Read the model definition and answer for the solid it produces. Units are mm, in the model's axes. A direction names the side the tool comes from. Give positions to 0.01 mm unless a question says otherwise; leave off trailing zeros. Write each loop counter-clockwise with the first axis right and the second up, starting at its lowest first coordinate (ties: lowest second). Pieces come first, ordered by that corner, then holes. Notation, with made-up numbers: M -5.5,-38 L 51.5,-38 A26 cw 51.5,-19 Z; hole C -25,10.25 d3. An arc over 180 degrees is marked long. Put each result on its own line as item: value.
from build123d import *

# Parameters (mm, degrees)
SKETCH2_W           = 38.1
SKETCH2_H           = 50.8
SKETCH2_R           = 13.335
BOSS_EXTRUDE2_DEPTH = 3.175
SKETCH4_W           = 38.1
SKETCH4_H           = 50.8
SKETCH4_R           = 13.335
BOSS_EXTRUDE3_DEPTH = 3.175
BOSS_EXTRUDE4_DEPTH = 127
CUT_EXTRUDE3_DEPTH  = 127
BOSS_EXTRUDE7_DEPTH = 127
SKETCH16_R          = 38.1
BOSS_EXTRUDE8_DEPTH = 25.4
CUT_EXTRUDE6_REACH  = 522.886
SKETCH19_W          = 33.866666667
SKETCH19_H          = 115.824
SKETCH19_W_2        = 33.866666666
CUT_EXTRUDE7_DEPTH  = 34.925


with BuildPart() as part:
    # Sketch2 → Boss-Extrude2 (new, symmetric)
    with BuildSketch(Plane(origin=(63.5, 0, 0), x_dir=(0, 0, -1), z_dir=(1, 0, 0))):
        Rectangle(SKETCH2_W, SKETCH2_H)
        Circle(SKETCH2_R, mode=Mode.SUBTRACT)
    extrude(amount=BOSS_EXTRUDE2_DEPTH, both=True)



with BuildPart() as body_2:
    # Sketch4 → Boss-Extrude3 (new, symmetric)
    with BuildSketch(Plane(origin=(292.1, 0, -263.652), x_dir=(0, 0, 1), z_dir=(-1, 0, 0))):
        with Locations((263.652, 0)):
            Rectangle(SKETCH4_W, SKETCH4_H)
        with Locations(Location((263.652, 0, 0), (0, 0, 180))):
            Circle(SKETCH4_R, mode=Mode.SUBTRACT)
    extrude(amount=BOSS_EXTRUDE3_DEPTH, both=True)


with BuildPart() as part_1:
    add(part.part)

    add(body_2.part)  # Boss-Extrude4 merges body 2
    # Sketch6 → Boss-Extrude4 (add, symmetric)
    with BuildSketch(Plane(origin=(177.8, 0, 0), x_dir=(0, 0, -1), z_dir=(1, 0, 0))):
        Polygon((-19.05, -25.4), (-61.976, -25.4), (-61.976, -255.524), (236.474, -255.524), (236.474, -217.424), (134.874, -25.4), (19.05, -25.4), align=None)
    extrude(amount=BOSS_EXTRUDE4_DEPTH, both=True)

    # Sketch13 → Cut-Extrude3 (cut, symmetric)
    with BuildSketch(Plane(origin=(177.8, 0, 0), x_dir=(0, 0, -1), z_dir=(1, 0, 0))):
        Polygon((-52.451, -34.925), (129.137596743, -34.925), (226.949, -219.788552156), (226.949, -255.524), (-61.976, -255.524), (-61.976, -219.788552156), (-52.451, -219.788552156), align=None)
    extrude(amount=CUT_EXTRUDE3_DEPTH, both=True, mode=Mode.SUBTRACT)

    # Sketch14 → Boss-Extrude7 (add, symmetric)
    with BuildSketch(Plane(origin=(177.8, 0, 0), x_dir=(0, 0, -1), z_dir=(1, 0, 0))):
        Polygon((226.949, -219.788552156), (-52.451, -219.788552156), (-52.451, -210.263552156), (221.90931746, -210.263552156), align=None)
        Polygon((-52.451, -146.763552156), (188.311433862, -146.763552156), (183.271751323, -137.238552156), (-52.451, -137.238552156), align=None)
    extrude(amount=BOSS_EXTRUDE7_DEPTH, both=True)

    # Sketch16 → Boss-Extrude8 (add)
    with BuildSketch(Plane(origin=(304.8, 0, 0), x_dir=(0, 0, -1), z_dir=(1, 0, 0))):
        with Locations(Location((-23.876, -232.488552156, 0), (0, 0, 160.528779366))):
            Circle(SKETCH16_R)
        with Locations(Location((160.274, -232.488552156, 0), (0, 0, 160.528779366))):
            Circle(SKETCH16_R)
    boss_extrude8 = extrude(amount=BOSS_EXTRUDE8_DEPTH)

    # Mirror1: Boss-Extrude8 across plane
    add(boss_extrude8.mirror(Plane(origin=(177.8, 0, 0), x_dir=(0, 0, 1), z_dir=(1, 0, 0))))

    # Cut-Extrude6: up to this plane
    cut_extrude6_end = Plane(origin=(50.8, -34.925, -129.137596743), z_dir=(0, 0.46767282988430103, -0.8839016484813284))
    # Sketch19 → Cut-Extrude6 (cut, up to the surface)
    with BuildSketch(Plane(origin=(0, 0, -236.474), x_dir=(-1, 0, 0), z_dir=(0, 0, -1)), mode=Mode.PRIVATE) as cut_extrude6_sk1:
        with Locations((-249.766666666, -121.412)):
            Rectangle(SKETCH19_W, SKETCH19_H)
    cut_extrude6_tool1 = split(extrude(cut_extrude6_sk1.sketch, amount=-CUT_EXTRUDE6_REACH, mode=Mode.PRIVATE), bisect_by=cut_extrude6_end, keep=Keep.BOTH, mode=Mode.PRIVATE)
    add(cut_extrude6_tool1.solids().sort_by_distance((249.766667, -121.412, -236.474))[0], mode=Mode.SUBTRACT)
    # Sketch19 → Cut-Extrude6 (cut, up to the surface)
    with BuildSketch(Plane(origin=(0, 0, -236.474), x_dir=(-1, 0, 0), z_dir=(0, 0, -1)), mode=Mode.PRIVATE) as cut_extrude6_sk2:
        with Locations((-177.8, -121.412)):
            Rectangle(SKETCH19_W_2, SKETCH19_H)
    cut_extrude6_tool2 = split(extrude(cut_extrude6_sk2.sketch, amount=-CUT_EXTRUDE6_REACH, mode=Mode.PRIVATE), bisect_by=cut_extrude6_end, keep=Keep.BOTH, mode=Mode.PRIVATE)
    add(cut_extrude6_tool2.solids().sort_by_distance((177.8, -121.412, -236.474))[0], mode=Mode.SUBTRACT)
    # Sketch19 → Cut-Extrude6 (cut, up to the surface)
    with BuildSketch(Plane(origin=(0, 0, -236.474), x_dir=(-1, 0, 0), z_dir=(0, 0, -1)), mode=Mode.PRIVATE) as cut_extrude6_sk3:
        with Locations((-105.833333334, -121.412)):
            Rectangle(SKETCH19_W, SKETCH19_H)
    cut_extrude6_tool3 = split(extrude(cut_extrude6_sk3.sketch, amount=-CUT_EXTRUDE6_REACH, mode=Mode.PRIVATE), bisect_by=cut_extrude6_end, keep=Keep.BOTH, mode=Mode.PRIVATE)
    add(cut_extrude6_tool3.solids().sort_by_distance((105.833333, -121.412, -236.474))[0], mode=Mode.SUBTRACT)

    # Sketch20 → Cut-Extrude7 (cut)
    with BuildSketch(Plane(origin=(0, 0, 0), x_dir=(1, 0, 0), z_dir=(0, 1, 0))):
        with BuildLine():
            Line((190.5, 93.599), (190.5, -20.701))
            ThreePointArc((190.5, -20.701), (177.8, -33.401), (165.1, -20.701))
            Line((165.1, -20.701), (165.1, 93.599))
            ThreePointArc((165.1, 93.599), (177.8, 106.299), (190.5, 93.599))
        make_face()
    extrude(amount=-CUT_EXTRUDE7_DEPTH, mode=Mode.SUBTRACT)


solid = part_1.part
(1) Section A-A on x = 177.8 is taken. Determine the outline of the cut face in (y, z) (3 decimals).
Result:
outline: M -255.524,-236.474 L -217.424,-236.474 L -179.324,-216.315 L -179.324,-205.539 L -210.264,-221.909 L -210.264,52.451 L -146.764,52.451 L -146.764,-188.311 L -137.239,-183.272 L -137.239,52.451 L -34.925,52.451 L -34.925,33.401 L -25.4,33.401 L -25.4,61.976 L -219.789,61.976 L -219.789,-226.949 L -255.524,-226.949 Z; M -63.5,-155.033 L -25.4,-134.874 L -25.4,-106.299 L -34.925,-106.299 L -34.925,-129.138 L -63.5,-144.257 Z
(2) Which of the six approach directions +Z, -Z, +X, -X, +Y, -Y give full straight-line access (tool end or side, diameter ignored) to faces 1 (the face through (50.8, -240, -158)), 2 (the face through (177.521, -30.096, -106.296)), 3 (the face through (50.8, -202, 27))?
Result:
face 1: +Z, -Y
face 2: +Y
face 3: none
(3) Section C-C on y = 0 is taken. Determine the outline of the cut face in (x, z) (3 decimals).
Result:
outline: M 60.325,-19.05 L 66.675,-19.05 L 66.675,-13.335 L 60.325,-13.335 Z; M 60.325,13.335 L 66.675,13.335 L 66.675,19.05 L 60.325,19.05 Z; M 288.925,-19.05 L 295.275,-19.05 L 295.275,-13.335 L 288.925,-13.335 Z; M 288.925,13.335 L 295.275,13.335 L 295.275,19.05 L 288.925,19.05 Z
(4) Section B-B on z = -31.5 is taken. Determine the outline of the cut face in (x, y) (3 decimals), and give its area (3 significant figures).
Result:
outline: M 50.8,-219.789 L 304.8,-219.789 L 304.8,-210.264 L 50.8,-210.264 Z; M 50.8,-146.764 L 304.8,-146.764 L 304.8,-137.239 L 50.8,-137.239 Z; M 50.8,-34.925 L 165.1,-34.925 L 165.1,-25.4 L 50.8,-25.4 Z; M 190.5,-34.925 L 304.8,-34.925 L 304.8,-25.4 L 190.5,-25.4 Z
area: 7,020 mm²
(5) Straight lines are drawn through the part: line 1 along Y through (x, z) = (65.25, 0) (3 decimals); line 2 along Y through (x, z) = (60.5, 29.5) (3 decimals); line 3 along Y through (x, z) = (98.5, -169.5). For each, find the intervals that lie inside material, in ascending order. Write a range as from..to.
Result:
line 1: y = -219.789..-210.264, -146.764..-137.239, -34.925..-13.335, 13.335..25.4
line 2: y = -219.789..-210.264, -146.764..-137.239, -34.925..-25.4
line 3: y = -219.79..-210.26, -146.76..-137.24
(6) Given pin 1 Ø12 at (x, z) = (258, -212.5) entering from +Y; pin 2 Ø1.5 at (x, z) = (89.5, -96.5) entering from +Y; pin 3 Ø1.9 at (x, y) = (292, -12) entering from +Z; pin 4 Ø24 at (y, z) = (0, 0) entering from +X, each flat-ended and moving along its own axis, determine where each tip first touches the part or whether it passes through.
Result:
pin 1: stops at y = -179.32
pin 2: stops at y = -25.4
pin 3: stops at z = 19.05
pin 4: passes through
(7) Section D-D on x = 210 is taken. Determine the outline of the cut face in (y, z) (3 decimals).
Result:
outline: M -255.524,-236.474 L -217.424,-236.474 L -25.4,-134.874 L -25.4,61.976 L -219.789,61.976 L -219.789,-226.949 L -255.524,-226.949 Z; hole M -210.264,-221.909 L -146.764,-188.311 L -146.764,52.451 L -210.264,52.451 Z; hole M -137.239,-183.272 L -34.925,-129.138 L -34.925,52.451 L -137.239,52.451 Z
(8) For a pull along Y with two mould halves and no side action, classify faces 4 (the face through (180, -87, 52.451)), 5 (the face through (66.675, 6, -12.4)), 6 (the face through (250, -179.324, -211)), 7 (the face through (180, -146.764, -66)) as +Y half, -Y half, draft (parallel to the pull), parting line (faces both ways), or undercut.
Result:
face 4: undercut
face 5: draft
face 6: +Y half
face 7: undercut
